Build history of the part. All positions in model axes, mm. Face numbers are marked on the shaded views. A direction names the side the tool comes from. Coordinates: 2 decimals unless noted, no trailing zeros. Loops run counter-clockwise (first coordinate to the right, second up) from the corner with the lowest first, then second, coordinate; pieces in that order, holes last.
Item 1: 3-axis set-ups, long thin cutter, end or side, ignore diameter. For the marked faces 1, 2 and 3: which of +Z, -Z, +X, -X, +Y, -Y reach the whole face in a straight line?
Item 2: Drill centre lines: line 1 along X through (y, z) = (-14, 10); line 2 along Y through (x, z) = (41.5, 9); line 3 along X through (y, z) = (-1, 9.5). Where is each one in solid material? Low to high.
Item 3: Cut at A-A (z = 11). List the corners of the cut face in (x, y).
Item 4: Flat gauge pins, fed straight in: pin 1 (4 mm diameter, centred on y = -1, z = 9.5, fed in from -X); pin 2 (9 mm diameter, centred on x = 43.5, z = 11.5, fed in from +Y); pin 3 (3 mm diameter, centred on x = -41.5, y = -14, fed in from +Z); pin 4 (2 mm diameter, centred on y = 3, z = 12, fed in from +X). Where does each tip first touch, or does it go through?
Item 5: Mould opens along X. For the marked faces 4, 5 and 6 say: released by +X, released by -X, zero draft, split by the parting line, or undercut.
Item 6: Cut at B-B (x = 41.5). List the corners of the cut face in (y, z), and give its area (3 significant figures).
Item 7: Cut at C-C (y = -14). List the corners of the cut face in (x, z).
Item 8: Cut at D-D (z = 15.75). List the corners of the cut face in (x, y), and give its area (3 significant figures).
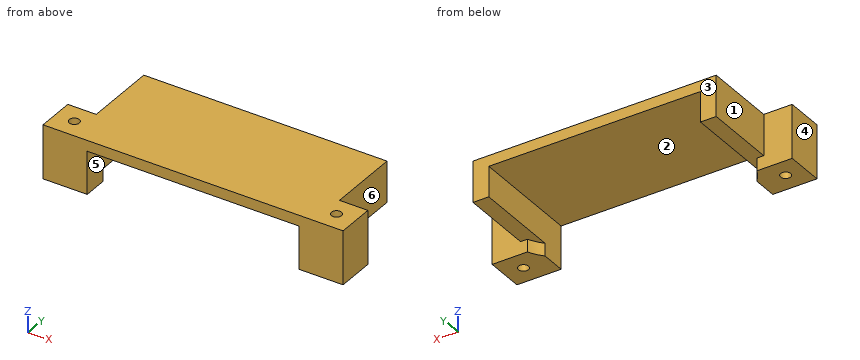
Autodesk Inventor part; units mm, degrees
ref_plane "Plano de trabajo1" through (-47.5, -94.8095, 26) normal (0, 0, 1) x (1, 0.0000001, 0)
ref_plane "YZ Plane" through (0, 0, 0) normal (1, 0, 0) x (0, 1, 0)
ref_plane "XZ Plane" through (0, 0, 0) normal (0, 1, 0) x (-1, 0, 0)
sketch "Boceto1" plane through (0, 0, 0) normal (0, 0, 1) x (1, 0, 0)
  line L0 (9.8963, 1.0011) -> (-9.8944, 1.0011)
  arc A0 (-33.0611, -12.6806) -> (-9.8944, 1.0011) centre (-23.4499, -2.5004) ccw
  line L1 (-33.0611, -12.6806) -> (-33.2, -12.6806)
  line L2 (-33.2, -12.6806) -> (-33.2, -12.5477)
  arc A1 (-37.0054, 1.0011) -> (-33.2, -12.5477) centre (-23.4499, -2.5004) ccw
  line L3 (-37.0054, 1.0011) -> (-47.5, 1.0011)
  line L4 (-47.5, 1.0011) -> (-47.5, -20)
  line L5 (-47.5, -20) -> (47.5, -20)
  line L6 (47.5, -20) -> (47.5, 1.0011)
  line L7 (47.5, 1.0011) -> (37.0052, 1.0011)
  arc A2 (33.2, -12.5466) -> (37.0052, 1.0011) centre (23.4507, -2.5001) ccw
  line L8 (33.2, -12.5466) -> (33.2, -12.6806)
  line L9 (33.2, -12.6806) -> (33.06, -12.6806)
  arc A3 (9.8963, 1.0011) -> (33.06, -12.6806) centre (23.4507, -2.5001) ccw
  circle A4 centre (40.9504, -2.4989) radius 2.1
  circle A5 centre (5.9501, -2.5002) radius 2.1
  circle A6 centre (-5.9495, -2.4989) radius 2.1
  circle A7 centre (-40.9494, -2.4994) radius 2.1
  line L10 (47.5, -20) -> (41.5, -20)
  line L11 (41.5, -20) -> (41.5, -14)
  line L12 (41.5, -14) -> (47.5, -14)
  line L13 (47.5, -14) -> (47.5, -20)
  circle A8 centre (41.5, -14) radius 1.6
  line L14 (-47.5, -20) -> (-41.5, -20)
  line L15 (-41.5, -20) -> (-41.5, -14)
  line L16 (-41.5, -14) -> (-47.5, -14)
  line L17 (-47.5, -14) -> (-47.5, -20)
  circle A9 centre (-41.5, -14) radius 1.6
  line L18 (47.5, -20) -> (33.5, -20)
  line L19 (33.5, -20) -> (33.5, -8)
  line L20 (33.5, -8) -> (47.5, -8)
  line L21 (47.5, -8) -> (47.5, -20)
  line L22 (-47.5, -20) -> (-33.5, -20)
  line L23 (-33.5, -20) -> (-33.5, -8)
  line L24 (-33.5, -8) -> (-47.5, -8)
  line L25 (-47.5, -8) -> (-47.5, -20)
  line L26 (33.2, -20.6806) -> (-33.2, -20.6806)
  line L27 (33.2, -12.6806) -> (33.2, -20.6806)
  line L28 (33.2, -12.6806) -> (30.95, -12.6806)
  arc A10 (25.95, -17.6806) -> (30.95, -12.6806) centre (25.95, -12.6806) ccw
  line L29 (25.95, -17.6806) -> (-25.95, -17.6806)
  arc A11 (-30.95, -12.6806) -> (-25.95, -17.6806) centre (-25.95, -12.6806) ccw
  line L30 (-33.2, -12.6806) -> (-30.95, -12.6806)
  line L31 (-33.2, -20.6806) -> (-33.2, -12.6806)
  line L32 (33.2, 62.3194) -> (33.2, -12.6806)
  line L33 (-33.2, -12.6806) -> (-33.2, 62.3194)
  circle A12 centre (-41.5, -14) radius 2.1
  circle A13 centre (41.5, -14) radius 2.1
  point P0 (0, 0)
  point P1 (47.5, -8)
  point P2 (33.5, -20)
  point P3 (-33.5, -20)
  point P4 (-47.5, -8)
  point P5 (-33.5, -12.2476)
  point P6 (-36.3249, -8)
  point P7 (36.3244, -8)
  point P8 (33.5, -12.2466)
  dimension "d0" = 6
  dimension "d1" = 6
  dimension "d2" = 3.2
  dimension "d3" = 6
  dimension "d4" = 6
  dimension "d5" = 3.2
  dimension "d6" = 14
  dimension "d7" = 12
  dimension "d8" = 14
  dimension "d9" = 12
ref_plane "Plano de trabajo1" through (-47.5, -94.8095, 26) normal (0, 0, 1) x (1, 0.0000001, 0)
extrude "Extrusión1" add sketch "Boceto1" along normal blind 17 contours A2 L20 L6 L12 A13 L11 L5 L19 | L23 L5 L15 A12 L16 L4 L24 A1 | L11 A13 L12 L6 L5 | L5 L4 L16 A12 L15 | A13 L12 A8 L11 | L11 A8 L12 A13 | A12 L16 A9 L15 | L15 A9 L16 A12
sketch "Boceto2" plane through (33.5, -20, 0) normal (-1, 0, 0) x (0, 0, 1)
  line L0 (0, 7.7534) -> (0, 0)
  line L1 (0, 0) -> (17, 0)
  line L2 (17, 7.7534) -> (17, 0)
  line L3 (0, 7.7534) -> (17, 7.7534)
  line L4 (13, 7.3194) -> (13, -0.6806)
  line L5 (13.6, 7.7534) -> (13.6, -0.6806)
  line L6 (0, 12) -> (0, 7.7534)
  line L7 (0, 7.7534) -> (17, 7.7534)
  line L8 (17, 12) -> (17, 7.7534)
  line L9 (0, 12) -> (17, 12)
  line L10 (13.6, 0) -> (17, 0)
  line L11 (17, 0) -> (17, 35)
  line L12 (17, 35) -> (13.6, 35)
  line L13 (13.6, 35) -> (13.6, 0)
  point P0 (0, 20)
  point P1 (17, 7.7534)
  point P2 (17, 12)
  point P3 (13.6, 12)
  point P4 (17, 12)
  point P5 (0, 7.7534)
  point P6 (17, 7.7534)
  point P7 (17, 7.7534)
  point P8 (13.6, 7.7534)
  point P9 (0, 7.7534)
  point P10 (17, 7.7534)
  point P11 (0, 7.7534)
  dimension "d12" = 0.6
  dimension "d13" = 35
extrude "Extrusión2" add sketch "Boceto2" along normal blind 72 and the other way blind 5 contours L13 L9 L8 L3 | L3 L2 L1 L5 | L13 L12 L11 L9
sketch "Boceto3" plane through (33.5, -20, 13.6) normal (0, 0, -1) x (-1, 0, 0)
  line L0 (67, 7.7524) -> (67, 0)
  arc A0 (67, 7.7524) -> (69.8249, 12) centre (56.9499, 17.4996) ccw
  line L1 (72, 12) -> (69.8249, 12)
  line L2 (72, 35) -> (72, 12)
  line L3 (72, 35) -> (-5, 35)
  line L4 (-5, 12) -> (-5, 35)
  line L5 (-2.8244, 12) -> (-5, 12)
  arc A1 (-2.8244, 12) -> (0, 7.7534) centre (10.0493, 17.4999) ccw
  line L6 (0, 0) -> (0, 7.7534)
  line L7 (0, 0) -> (67, 0)
  line L8 (0.3, 7.3194) -> (0.3, 82.3194)
  line L9 (0, 7.7534) -> (0.3, 7.7534)
  line L10 (66.7, 7.3194) -> (66.7, 82.3194)
  line L11 (67, 7.7524) -> (67, 0)
  line L12 (67, 7.7524) -> (67, 36)
  line L13 (0, 7.7534) -> (0, 35.331)
  point P0 (33.5, 20)
  point P1 (0.3, 35)
  point P2 (67, 35)
  point P3 (0, 35)
extrude "Extrusión3" add sketch "Boceto3" along normal blind 9.6 contours L12 L3 L2 L1 A0 | A1 L5 L4 L3 L13
properties part number "Tapadera cremallera"
Filled sheet:
1. face 1: +Z, -Z, -X, +Y
1. face 2: -Z, +Y, -Y
1. face 3: +Z, -Z, +X, -X, +Y
2. line 1: x = -47.5 to -43.1, -39.9 to -33.5, 33.5 to 39.9, 43.1 to 47.5
2. line 2: y = -20 to -15.6, -12.4 to -8
2. line 3: x = -38.5 to -33.5, 33.5 to 38.5
3. outline: (-47.5, -20) - (-33.5, -20) - (-33.5, 15) - (-38.5, 15) - (-38.5, -8) - (-47.5, -8) - close; (33.5, -20) - (47.5, -20) - (47.5, -8) - (38.5, -8) - (38.5, 15) - (33.5, 15) - close; hole circle Ø3.2 at (-41.5, -14); hole circle Ø3.2 at (41.5, -14)
4. pin 1: stops at x = -38.5
4. pin 2: stops at y = -8
4. pin 3: passes through
4. pin 4: stops at x = 38.5
5. face 4: released by -X
5. face 5: undercut
5. face 6: released by +X
6. outline: (-20, 0) - (-15.6, 0) - (-15.6, 17) - (-20, 17) - close; (-12.4, 0) - (-8, 0) - (-8, 17) - (-12.4, 17) - close
6. area: 150 mm2
7. outline: (-47.5, 0) - (-43.1, 0) - (-43.1, 17) - (-47.5, 17) - close; (-39.9, 0) - (-33.5, 0) - (-33.5, 13.6) - (33.5, 13.6) - (33.5, 0) - (39.9, 0) - (39.9, 17) - (-39.9, 17) - close; (43.1, 0) - (47.5, 0) - (47.5, 17) - (43.1, 17) - close
8. outline: (-47.5, -20) - (47.5, -20) - (47.5, -8) - (38.5, -8) - (38.5, 15) - (-38.5, 15) - (-38.5, -8) - (-47.5, -8) - close; hole circle Ø3.2 at (-41.5, -14); hole circle Ø3.2 at (41.5, -14)
8. area: 2,890 mm2
